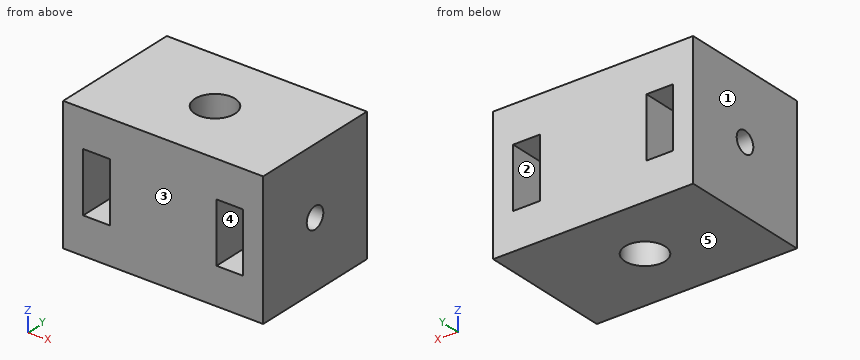
```python
from build123d import *

# Parameters (mm, degrees)
F0_W     = 15
F0_H     = 10
F1_DEPTH = 10
F2_W     = 2
F2_H     = 4.5
F3_DEPTH = 10
F4_R     = 1.5
F5_DEPTH = 15
F6_R     = 0.8
F7_DEPTH = 15


with BuildPart() as f1:
    # F0 (on Top) → F1 (new body)
    with BuildSketch(Plane.XY):
        Rectangle(F0_W, F0_H)
    extrude(amount=F1_DEPTH)

    # F2 (on face) → F3 (cut, through all)
    with BuildSketch(Plane.XZ.offset(5)):
        with Locations((-5, 5)):
            Rectangle(F2_W, F2_H)
        with Locations((5, 5)):
            Rectangle(F2_W, F2_H)
    extrude(amount=-F3_DEPTH, mode=Mode.SUBTRACT)

    # F4 (on face) → F5 (cut)
    with BuildSketch(Plane(origin=(0, 0, 0), x_dir=(1, 0, 0), z_dir=(0, 0, -1))):
        Circle(F4_R)
    extrude(amount=-F5_DEPTH, mode=Mode.SUBTRACT)

    # F6 (on face) → F7 (cut, through all)
    with BuildSketch(Plane(origin=(-7.5, 0, 0), x_dir=(0, -1, 0), z_dir=(-1, 0, 0))):
        with Locations((0, 5)):
            Circle(F6_R)
    extrude(amount=-F7_DEPTH, mode=Mode.SUBTRACT)


solid = f1.part
```
Source: CAD feature listing. Evaluate the final solid. Frame: model axes, mm. Face numbers are marked on the shaded views. A direction names the side the tool comes from. Give positions to 0.01 mm unless a question says otherwise; leave off trailing zeros. Order: outer loops, then holes, each group sorted by start corner. A loop starts at its lowest first (then second) coordinate and runs counter-clockwise, first axis right, second up. Notation, with made-up numbers: (65, -35.75) -> (109, -35.75) arc R18 cw to (109, -9.75) -> close; hole circle Ø1 at (60.25, 56.25). An arc over 180 degrees is marked (long way). Use a Markdown table: item, result.
Q1. Section A-A (z = 3). Return the cut outline in (x, y).
A:
| item | result |
|---|---|
| outline | (-7.5, -5) -> (-6, -5) -> (-6, 5) -> (-7.5, 5) -> close; (-4, -5) -> (4, -5) -> (4, 5) -> (-4, 5) -> close; (6, -5) -> (7.5, -5) -> (7.5, 5) -> (6, 5) -> close; hole circle Ø3 at (0, 0) |
Q2. Section C-C (z = 5). Return the cut outline in (x, y).
A:
| item | result |
|---|---|
| outline | (-7.5, -5) -> (-6, -5) -> (-6, -0.8) -> (-7.5, -0.8) -> close; (-7.5, 0.8) -> (-6, 0.8) -> (-6, 5) -> (-7.5, 5) -> close; (-4, -5) -> (4, -5) -> (4, -0.8) -> (1.27, -0.8) arc R1.5 cw to (-1.27, -0.8) -> (-4, -0.8) -> close; (-4, 0.8) -> (-1.27, 0.8) arc R1.5 cw to (1.27, 0.8) -> (4, 0.8) -> (4, 5) -> (-4, 5) -> close; (6, -5) -> (7.5, -5) -> (7.5, -0.8) -> (6, -0.8) -> close; (6, 0.8) -> (7.5, 0.8) -> (7.5, 5) -> (6, 5) -> close |
Q3. Access query for the marked faces 1 and 2. Directions: +Z, -Z, +X, -X, +Y, -Y. A direction counts if a zero-diameter tool reaches every point of the face in a straight line with its end or side. Return the directions, or none.
A:
| item | result |
|---|---|
| face 1 | +Z, -Z, -X, +Y, -Y |
| face 2 | +Y, -Y |
Q4. Section D-D (x = 0). Return the cut outline in (y, z).
A:
| item | result |
|---|---|
| outline | (-5, 0) -> (-1.5, 0) -> (-1.5, 10) -> (-5, 10) -> close; (1.5, 0) -> (5, 0) -> (5, 10) -> (1.5, 10) -> close |
Q5. Section B-B (y = 0). State how many separate pieces and enclosed holes the cut face has, and give its area (3 significant figures).
A:
| item | result |
|---|---|
| separate pieces | 4 |
| enclosed holes | 0 |
| area | 89.2 mm^2 |
Q6. Pull-direction query (Z, two-part tool) for the marked faces 3, 4 and 5; classes: +Z half, -Z half, draft (parallel to the pull), parting line (faces both ways), or undercut.
A:
| item | result |
|---|---|
| face 3 | draft |
| face 4 | undercut |
| face 5 | -Z half |
Q7. Material intervals for line 1 (X direction, y = 1.75, z = 5); line 2 (X direction, y = 0, z = 6.75); line 3 (Z direction, x = -2.25, y = 0), sorted ascending. Write a range as [from, to].
A:
| item | result |
|---|---|
| line 1 | [-7.5, -6], [-4, 4], [6, 7.5] |
| line 2 | [-7.5, -6], [-4, -1.5], [1.5, 4], [6, 7.5] |
| line 3 | [0, 4.2], [5.8, 10] |
